For this review, take the finished solid that the model builds, in its own axes (mm). A direction names the side the tool comes from. Give positions to 0.01 mm unless a question says otherwise; leave off trailing zeros. Loops run counter-clockwise (first coordinate to the right, second up) from the corner with the lowest first, then second, coordinate; pieces in that order, holes last. Notation, with made-up numbers: (59.25, 15) - (97.25, 15) arc R21 cw to (97.25, 38) - close; hole circle Ø5 at (-30, -8.5). An arc over 180 degrees is marked (long way). Answer in a Markdown table with one row per item.
```python
from build123d import *

# Parameters (mm, degrees)
F0_R     = 50.8
F2_R     = 19.05
F4_R     = 19.05
F5_DEPTH = 50.8
F6_T     = -2.54


with BuildPart() as f3:
    # F0 (on Top) → F3 section 0
    with BuildSketch(Plane.XY):
        Circle(F0_R)
    # F2 (on offset) → F3 section 1
    with BuildSketch(Plane.XY.offset(76.2)):
        Circle(F2_R)
    loft()

    # F4 (on face) → F5 (join)
    with BuildSketch(Plane.XY.offset(76.2)):
        Circle(F4_R)
    extrude(amount=F5_DEPTH)

    # F6
    f6_openings = [f3.faces().sort_by_distance(p)[0] for p in [
        (0, 0, 127),
    ]]
    offset(amount=F6_T, openings=f6_openings, kind=Kind.INTERSECTION)


solid = f3.part
```
1. Wall thickness on line 1 (Y direction, x = 0, z = 95); line 2 (Z direction, x = -1, y = -6); line 3 (X direction, y = -35, z = 7.5): over which ranges is each line inside the solid? List them lowest first. Write a range as [from, to].
Values:
| item | result |
|---|---|
| line 1 | y = [-19.05, -16.51], [16.51, 19.05] |
| line 2 | z = [0, 2.54] |
| line 3 | x = [-32.37, -28.16], [28.16, 32.37] |
2. We need section C-C, the plane z = 55. Give the boundary of the cut face in (x, y).
Values:
| item | result |
|---|---|
| outline | circle Ø55.77 at (0, 0); hole circle Ø50.26 at (0, 0) |
3. Mouldability with a two-part tool opening along X and no side actions: class faces 4 (the face through (-4.06, 30.91, 47.1)), 5 (the face through (15.748, 4.959, 100.987)), 6 (the face through (-1, 1, 0)) as released by +X, released by -X, zero draft, split by the parting line, or undercut.
Values:
| item | result |
|---|---|
| face 4 | split by the parting line |
| face 5 | undercut |
| face 6 | zero draft |
4. For faces 1 (the face through (-15.12, -11.59, 101.24)), 2 (the face through (-6, 16, 127)), 3 (the face through (12.99, -24.97, 47.76)), list the 3-axis set-ups (+Z, -Z, +X, -X, +Y, -Y) from which the entire face can be reached by the end or side of a thin tool; tool diameter is ignored.
Values:
| item | result |
|---|---|
| face 1 | +Z |
| face 2 | +Z, +X, -X, +Y, -Y |
| face 3 | none |
5. Clearance check with flat-ended pins moving along their axes: pin 1 (12 mm diameter, centred on x = -0.5, z = 46, fed in from +Y); pin 2 (3 mm diameter, centred on x = -19.5, z = 58, fed in from -Y); pin 3 (8 mm diameter, centred on x = 30, z = 20, fed in from +Y). State where each tip first meets the part, or that it passes through.
Values:
| item | result |
|---|---|
| pin 1 | stops at y = 34.13 |
| pin 2 | stops at y = -19.87 |
| pin 3 | stops at y = 34.23 |
6. We need section A-A, the plane x = 0. Give the boundary of the cut face in (y, z), and give its area (3 significant figures).
Values:
| item | result |
|---|---|
| outline | (-50.8, 0) - (50.8, 0) - (19.05, 76.2) - (19.05, 127) - (16.51, 127) - (16.51, 75.69) - (46.99, 2.54) - (-46.99, 2.54) - (-16.51, 75.69) - (-16.51, 127) - (-19.05, 127) - (-19.05, 76.2) - close |
| area | 919 mm^2 |
7. We need section B-B, the plane z = 23.5. Give the boundary of the cut face in (x, y).
Values:
| item | result |
|---|---|
| outline | circle Ø82.02 at (0, 0); hole circle Ø76.51 at (0, 0) |
